Study the drawing (mm; zero at the part's minimum x, y, z) and answer. Round coordinates to 2 decimals unless told otherwise and drop trailing zeros. Order: outer loops, then holes, each group sorted by start corner. A loop starts at its lowest first (then second) coordinate and runs counter-clockwise, first axis right, second up. Notation, with made-up numbers: (-40, -5.75) - (-29, -5.75) arc R14 ccw to (-29, 0.25) - close; hole circle Ø1 at (61, 65). An arc over 180 degrees is marked (long way). Put each result on its own line as item: value. Start each with the question number.
Q1. Find the intervals of material crossed by line 1 along Z through (x, y) = (12.5, 1.05); line 2 along X through (y, z) = (1.75, 3); line 3 along Z through (x, y) = (21.25, 2.85), in increasing order. Write a range as from..to.
Q2. Section A-A on x = 12.5 is taken. Give the vertices of the cut face in (y, z), then the cut area to 3 significant figures.
Q3. Each of these flat-tipped pins is pushed along its axis until it touches: pin 1 Ø1.5 at (x, y) = (3.5, 1.5) entering from +Z; pin 2 Ø1.6 at (y, z) = (1, 58.5) entering from -X; pin 3 Ø1 at (y, z) = (1, 58) entering from +X. Where does it stop, or does it pass through?
Q4. Section B-B on y = 1.05 is taken. Give the vertices of the cut face in (x, z) (3 decimals), then the cut area to 3 significant figures.
Q5. Section D-D on x = 18.5 is taken. Give the vertices of the cut face in (y, z).
Q6. Section C-C on z = 6.5 is taken. Give the vertices of the cut face in (x, y), then the cut area to 3 significant figures.
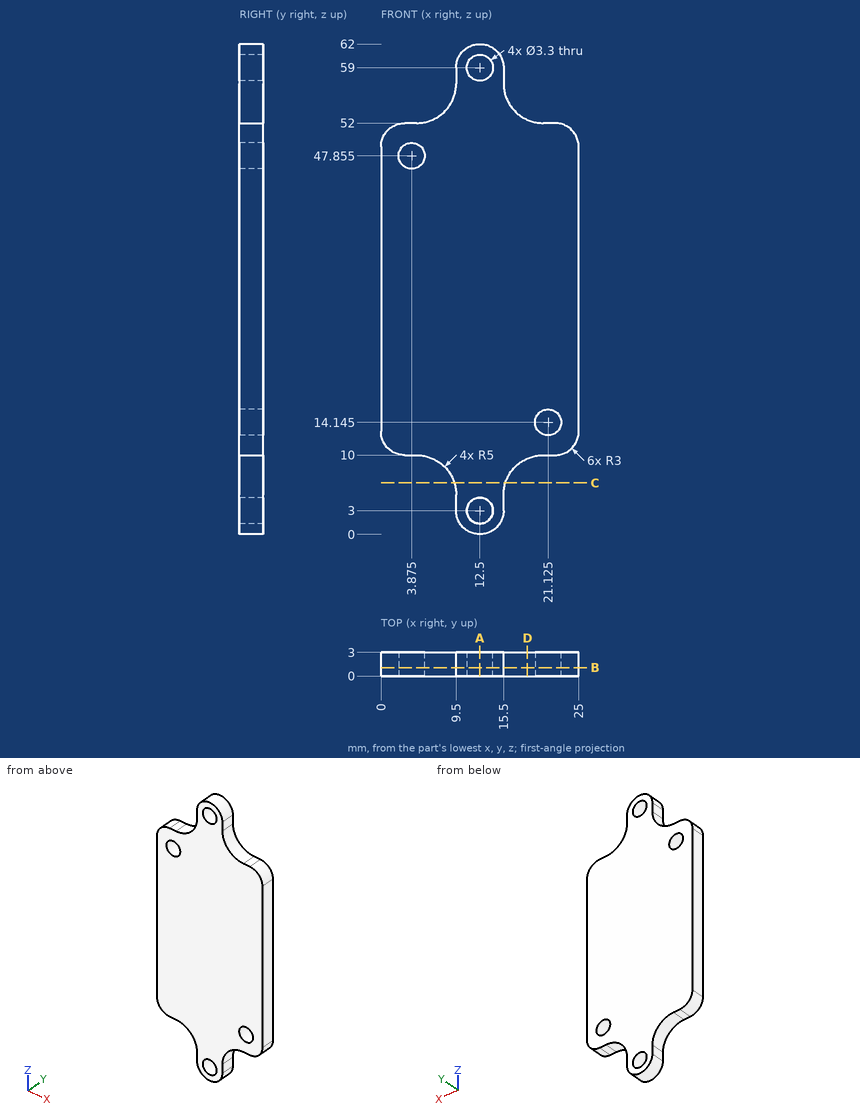
Findings:
1. line 1: 0..1.35, 4.65..57.35, 60.65..62
1. line 2: 9.5..10.85, 14.15..15.5
1. line 3: 10..12.5, 15.79..52
2. outline: (0, 0) - (3, 0) - (3, 1.35) - (0, 1.35) - close; (0, 4.65) - (3, 4.65) - (3, 57.35) - (0, 57.35) - close; (0, 60.65) - (3, 60.65) - (3, 62) - (0, 62) - close
2. area: 166 mm2
3. pin 1: z = 52
3. pin 2: x = 9.5
3. pin 3: x = 15.5
4. outline: (0, 13) arc R3 ccw to (3, 10) - (4.5, 10) arc R5 cw to (9.5, 5) - (9.5, 3) arc R3 ccw to (15.5, 3) - (15.5, 5) arc R5 cw to (20.5, 10) - (22, 10) arc R3 ccw to (25, 13) - (25, 49) arc R3 ccw to (22, 52) - (20.5, 52) arc R5 cw to (15.5, 57) - (15.5, 59) arc R3 ccw to (9.5, 59) - (9.5, 57) arc R5 cw to (4.5, 52) - (3, 52) arc R3 ccw to (0, 49) - close; hole circle Ø3.3 at (3.875, 47.855); hole circle Ø3.3 at (12.5, 3); hole circle Ø3.3 at (12.5, 59); hole circle Ø3.3 at (21.125, 14.145)
4. area: 1,140 mm2
5. outline: (0, 9.58) - (3, 9.58) - (3, 52.42) - (0, 52.42) - close
6. outline: (9.27, 0) - (15.73, 0) - (15.73, 3) - (9.27, 3) - close
6. area: 19.4 mm2
